Input: part model. Units: mm. Frame: model coordinates. A direction names the side the tool comes from. Round coordinates to 2 decimals unless told otherwise and drop trailing zeros. Loops run counter-clockwise (first coordinate to the right, second up) from the corner with the lowest first, then second, coordinate; pieces in that order, holes last. Notation, with made-up numbers: (33.5, 58.25) -> (77.5, 58.25) arc R19 ccw to (77.5, 93.25) -> close; hole circle Ø3 at (-2, 75.25). An arc over 180 degrees is marked (long way). Answer as a JSON object with one key per item and string values.
Autodesk Inventor part; units mm, degrees
ref_plane "YZ Plane" through (0, 0, 0) normal (1, 0, 0) x (0, 1, 0)
ref_plane "XZ Plane" through (0, 0, 0) normal (0, 1, 0) x (-1, 0, 0)
ref_plane "XY Plane" through (0, 0, 0) normal (0, 0, 1) x (1, 0, 0)
sketch "Sketch2" plane through (0, 0, 0) normal (0, 1, 0) x (-1, 0, 0)
  circle A0 centre (0, 0) radius 3.52 construction
  circle A1 centre (0, 0) radius 2.3784 construction
  line L0 (-4, 4) -> (4, 4) construction
  line L1 (4, 4) -> (4, -4) construction
  line L2 (-0.8, 2.2399) -> (-0.8, 0.8)
  line L3 (-0.8, 0.8) -> (-2.2399, 0.8)
  line L4 (-2.2399, -0.8) -> (-0.8, -0.8)
  line L5 (-0.8, -0.8) -> (-0.8, -2.2399)
  line L6 (0.8, -2.2399) -> (0.8, -0.8)
  line L7 (0.8, -0.8) -> (2.2399, -0.8)
  line L8 (2.2399, 0.8) -> (0.8, 0.8)
  line L9 (0.8, 0.8) -> (0.8, 2.2399)
  arc A2 (0.8, 2.2399) -> (-0.8, 2.2399) centre (0, 0) ccw
  arc A3 (-2.2399, 0.8) -> (-2.2399, -0.8) centre (0, 0) ccw
  arc A4 (-0.8, -2.2399) -> (0.8, -2.2399) centre (0, 0) ccw
  arc A5 (2.2399, -0.8) -> (2.2399, 0.8) centre (0, 0) ccw
  circle A6 centre (-4, 4) radius 2.4
  circle A7 centre (4, 4) radius 2.4
  circle A8 centre (-4, -4) radius 2.4
  circle A9 centre (4, -4) radius 2.4
  arc A10 (1.6845, 3.3686) -> (-1.6845, 3.3686) centre (0, -5.93) ccw
  line L10 (-3.4, 1.6762) -> (-3.4, -1.6762)
  line L11 (3.4, 1.6762) -> (3.4, -1.6762)
  arc A11 (-1.6845, -3.3686) -> (1.6845, -3.3686) centre (0, 5.93) ccw
  circle A12 centre (0, 0) radius 1.1314
  point P0 (0, 4)
  point P1 (4, 0)
  dimension "d0" = 4.7569
  dimension "d1" = 7.04
  dimension "d2" = 8
  dimension "d4" = 1.6
  dimension "d20" = 4.8
  dimension "d21" = 18.9
  dimension "d22" = 6.8
extrude "Extrusion1" add sketch "Sketch2" along normal mid plane 16 contours A6 A10 A7 L11 A9 A11 A8 L10
extrude "Extrusion3" add sketch "Sketch2" along normal mid plane 0.2 contours A2 L9 A12 L2 | A12 L4 A3 L3 | L8 A5 L7 A12 | A12 L6 A4 L5
fillet "Fillet1" radius 0.1 24 edges at (1.6845, 0, 3.3686) (3.4, 0, 1.6762) (-1.6845, 0, 3.3686) (-3.4, 0, 1.6762) (3.4, 0, -1.6762) (1.6845, 0, -3.3686) (-1.6845, 0, -3.3686) (-3.4, 0, -1.6762) (2.3145, 8, 2.2915) (0, 8, 3.52) (-2.3145, 8, 2.2915) (-3.4, 8, 0) (-2.3145, 8, -2.2915) (0, 8, -3.52) (2.3145, 8, -2.2915) (3.4, 8, 0) (3.4, -8, 0) (2.3145, -8, 2.2915) (0, -8, 3.52) (-2.3145, -8, 2.2915) (-3.4, -8, 0) (-2.3145, -8, -2.2915) (0, -8, -3.52) (2.3145, -8, -2.2915)
equation "\"d2\" = lu"
equation "\"d4\" = axlet"
properties part number "6538c-White" material "ABS Plastic"
1) Section B-B, the plane x = 0. Output: boundary loops of the cut face in (y, z), plus the area to 3 significant figures.
Output:
{"outline": "(-8, -3.42) arc R0.1 ccw to (-7.9, -3.52) -> (7.9, -3.52) arc R0.1 ccw to (8, -3.42) -> (8, -2.38) -> (0.1, -2.38) -> (0.1, -1.13) -> (-0.1, -1.13) -> (-0.1, -2.38) -> (-8, -2.38) -> close; (-8, 2.38) -> (-0.1, 2.38) -> (-0.1, 1.13) -> (0.1, 1.13) -> (0.1, 2.38) -> (8, 2.38) -> (8, 3.42) arc R0.1 ccw to (7.9, 3.52) -> (-7.9, 3.52) arc R0.1 ccw to (-8, 3.42) -> close", "area": "37.0 mm^2"}
2) Contact query for flat-ended pins moving along their axis: P1, Ø1.2, axis at x = -1, y = 5.5, coming from the -Z side; P2, Ø0.8, axis at x = 0, z = -1.5, coming from the -Y side; P3, Ø1.6, axis at x = -2, y = -5.5, coming from the +Z side. Output: stop coordinate, or through.
Output:
{"P1": "stops at z = -3.51", "P2": "stops at y = -0.1", "P3": "stops at z = 3.44"}
3) Draft query along X for faces 4 (the face through (-2, -0.1, 0)), 5 (the face through (-1, -8, 1)), 6 (the face through (3.4, 0, 0)), 7 (the face through (-2, -4, 0.8)). Return one class per face: +X half, -X half, draft (parallel to the pull), parting line (faces both ways), or undercut.
Output:
{"face 4": "undercut", "face 5": "draft", "face 6": "+X half", "face 7": "undercut"}
4) Section A-A, the plane z = 0. Output: boundary loops of the cut face in (x, y), plus the area to 3 significant figures.
Output:
{"outline": "(-3.4, -7.9) arc R0.1 ccw to (-3.3, -8) -> (-2.38, -8) -> (-2.38, -0.1) -> (-1.13, -0.1) -> (-1.13, 0.1) -> (-2.38, 0.1) -> (-2.38, 8) -> (-3.3, 8) arc R0.1 ccw to (-3.4, 7.9) -> close; (1.13, -0.1) -> (2.38, -0.1) -> (2.38, -8) -> (3.3, -8) arc R0.1 ccw to (3.4, -7.9) -> (3.4, 7.9) arc R0.1 ccw to (3.3, 8) -> (2.38, 8) -> (2.38, 0.1) -> (1.13, 0.1) -> close", "area": "33.2 mm^2"}
5) Reachability of faces 1 (the face through (2.298, -0.111, 2.308)), 2 (the face through (2, 4, -0.8)), 3 (the face through (2, -4, 0.8)) from +Z, -Z, +X, -X, +Y, -Y: full face, straight path, thin tool, end or side. Return the list, or none.
Output:
{"face 1": "+Z, +X, +Y, -Y", "face 2": "+Y", "face 3": "-Y"}
6) Ray query, probe 1 along X at (y, z) = (0.05, 0); probe 2 along X at (y, z) = (1.5, -1.25); probe 3 along Y at (x, z) = (0, 1.5). Return the intervals inside material, ascending.
Output:
{"probe 1": "x = -3.4 to -1.13, 1.13 to 3.4", "probe 2": "x = -3.4 to -0.8, 0.8 to 3.4", "probe 3": "y = -0.1 to 0.1"}
